```python
from build123d import *

# Parameters (mm, degrees)
BOSS_EXTRUDE1_DEPTH = 165
SKETCH3_W           = 30
SKETCH3_H           = 32
BOSS_EXTRUDE2_DEPTH = 2
SKETCH4_W           = 30
SKETCH4_H           = 32
BOSS_EXTRUDE3_DEPTH = 2
BOSS_EXTRUDE4_START = 10
BOSS_EXTRUDE4_DEPTH = 10
CUT_EXTRUDE1_DEPTH  = 10
BOSS_EXTRUDE6_DEPTH = 15
CUT_EXTRUDE2_DEPTH  = 15
BOSS_EXTRUDE7_DEPTH = 121
CUT_EXTRUDE3_DEPTH  = 121
SKETCH13_W          = 169
SKETCH13_H          = 30
CUT_EXTRUDE5_DEPTH  = 3
SKETCH14_W          = 169
SKETCH14_H          = 30
BOSS_EXTRUDE8_DEPTH = 3
SKETCH12_W          = 28
SKETCH12_H          = 2
CUT_EXTRUDE6_DEPTH  = 168
SKETCH16_W          = 165
SKETCH16_H          = 26
CUT_EXTRUDE7_DEPTH  = 3
CUT_EXTRUDE8_DEPTH  = 1.5
CUT_EXTRUDE9_DEPTH  = 3
SKETCH20_W          = 169
SKETCH20_H          = 30
BOSS_EXTRUDE9_DEPTH = 1
SKETCH21_W          = 165
SKETCH21_H          = 26
CUT_EXTRUDE10_DEPTH = 1
FILLET1_START       = -16
FILLET1_DEPTH       = 35
FILLET1_2_DEPTH     = 32
FILLET2_R           = 1


with BuildPart() as part:
    # Sketch2 → Boss-Extrude1 (new body)
    with BuildSketch(Plane(origin=(0, 0, 0), x_dir=(0, 0, -1), z_dir=(1, 0, 0))):
        with BuildLine():
            Line((-13, 0), (-13, 17))
            Line((-13, 17), (-15, 17))
            Line((-15, 17), (-15, -15))
            Line((-15, -15), (15, -15))
            Line((15, -15), (15, 17))
            Line((15, 17), (13, 17))
            Line((13, 17), (13, 0))
            ThreePointArc((13, 0), (0, -13), (-13, 0))
        make_face()
    extrude(amount=BOSS_EXTRUDE1_DEPTH)

    # Sketch3 → Boss-Extrude2 (add)
    with BuildSketch(Plane(origin=(165, 0, 0), x_dir=(0, 0, -1), z_dir=(1, 0, 0))):
        with Locations((0, 1)):
            Rectangle(SKETCH3_W, SKETCH3_H)
    extrude(amount=BOSS_EXTRUDE2_DEPTH)

    # Sketch4 → Boss-Extrude3 (add)
    with BuildSketch(Plane.ZY):
        with Locations((0, 1)):
            Rectangle(SKETCH4_W, SKETCH4_H)
    extrude(amount=BOSS_EXTRUDE3_DEPTH)

    # Sketch5 → Boss-Extrude4 (add)
    with BuildSketch(Plane.ZY.offset(-165).offset(BOSS_EXTRUDE4_START)):
        with BuildLine():
            Line((-13, 17), (-13, 0))
            ThreePointArc((-13, 0), (0, -13), (13, 0))
            Line((13, 0), (13, 17))
            Line((13, 17), (-13, 17))
        make_face()
    extrude(amount=-BOSS_EXTRUDE4_DEPTH)

    # Sketch6 → Cut-Extrude1 (cut)
    with BuildSketch(Plane.ZY.offset(-155)):
        with BuildLine():
            Line((-2, 0), (-2, 17))
            Line((-2, 17), (2, 17))
            Line((2, 17), (2, 0))
            ThreePointArc((2, 0), (0, -2), (-2, 0))
        make_face()
    extrude(amount=-CUT_EXTRUDE1_DEPTH, mode=Mode.SUBTRACT)

    # Sketch8 → Boss-Extrude6 (add)
    with BuildSketch(Plane(origin=(0, 0, 0), x_dir=(0, 0, -1), z_dir=(1, 0, 0))):
        with BuildLine():
            Line((13, 0), (13, 17))
            Line((13, 17), (-13, 17))
            Line((-13, 17), (-13, 0))
            ThreePointArc((-13, 0), (0, -13), (13, 0))
        make_face()
    extrude(amount=BOSS_EXTRUDE6_DEPTH)

    # Sketch9 → Cut-Extrude2 (cut)
    with BuildSketch(Plane(origin=(15, 0, 0), x_dir=(0, 0, -1), z_dir=(1, 0, 0))):
        with BuildLine():
            Line((-2.125, 0), (-2.125, 17))
            Line((-2.125, 17), (2.125, 17))
            Line((2.125, 17), (2.125, 0))
            ThreePointArc((2.125, 0), (0, -2.125), (-2.125, 0))
        make_face()
    extrude(amount=-CUT_EXTRUDE2_DEPTH, mode=Mode.SUBTRACT)

    # Sketch10 → Boss-Extrude7 (add)
    with BuildSketch(Plane(origin=(15, 0, 0), x_dir=(0, 0, -1), z_dir=(1, 0, 0))):
        with BuildLine():
            Line((13, 0), (13, 17))
            Line((13, 17), (-13, 17))
            Line((-13, 17), (-13, 0))
            ThreePointArc((-13, 0), (0, -13), (13, 0))
        make_face()
    extrude(amount=BOSS_EXTRUDE7_DEPTH)

    # Sketch11 → Cut-Extrude3 (cut)
    with BuildSketch(Plane(origin=(136, 0, 0), x_dir=(0, 0, -1), z_dir=(1, 0, 0))):
        with BuildLine():
            Line((-8.5, 0), (-8.5, 17))
            Line((-8.5, 17), (8.5, 17))
            Line((8.5, 17), (8.5, 0))
            ThreePointArc((8.5, 0), (0, -8.5), (-8.5, 0))
        make_face()
    extrude(amount=-CUT_EXTRUDE3_DEPTH, mode=Mode.SUBTRACT)

    # Sketch13 → Cut-Extrude5 (cut)
    with BuildSketch(Plane(origin=(0, 17, 0), x_dir=(1, 0, 0), z_dir=(0, 1, 0))):
        with Locations((82.5, 0)):
            Rectangle(SKETCH13_W, SKETCH13_H)
    extrude(amount=-CUT_EXTRUDE5_DEPTH, mode=Mode.SUBTRACT)

    # Sketch14 → Boss-Extrude8 (add)
    with BuildSketch(Plane(origin=(0, 14, 0), x_dir=(1, 0, 0), z_dir=(0, 1, 0))):
        with Locations((82.5, 0)):
            Rectangle(SKETCH14_W, SKETCH14_H)
    extrude(amount=BOSS_EXTRUDE8_DEPTH)

    # Sketch12 → Cut-Extrude6 (cut)
    with BuildSketch(Plane(origin=(167, 0, 0), x_dir=(0, 0, -1), z_dir=(1, 0, 0))):
        with Locations((0, 15)):
            Rectangle(SKETCH12_W, SKETCH12_H)
    extrude(amount=-CUT_EXTRUDE6_DEPTH, mode=Mode.SUBTRACT)

    # Sketch16 → Cut-Extrude7 (cut)
    with BuildSketch(Plane(origin=(0, 17, 0), x_dir=(1, 0, 0), z_dir=(0, 1, 0))):
        with Locations((82.5, 0)):
            Rectangle(SKETCH16_W, SKETCH16_H)
    extrude(amount=-CUT_EXTRUDE7_DEPTH, mode=Mode.SUBTRACT)

    # Sketch17 → Cut-Extrude8 (cut)
    with BuildSketch(Plane(origin=(136, 0, 0), x_dir=(0, 0, -1), z_dir=(1, 0, 0))):
        with BuildLine():
            Line((13, 14), (13, 0))
            ThreePointArc((13, 0), (0, -13), (-13, 0))
            Line((-13, 0), (-13, 14))
            Line((-13, 14), (-8.5, 14))
            Line((-8.5, 14), (-8.5, 0))
            ThreePointArc((-8.5, 0), (0, -8.5), (8.5, 0))
            Line((8.5, 0), (8.5, 14))
            Line((8.5, 14), (13, 14))
        make_face()
    extrude(amount=-CUT_EXTRUDE8_DEPTH, mode=Mode.SUBTRACT)

    # Sketch18 → Cut-Extrude9 (cut)
    with BuildSketch(Plane(origin=(15, 0, 0), x_dir=(0, 0, -1), z_dir=(1, 0, 0))):
        with BuildLine():
            Line((8.5, 0), (8.5, 14))
            Line((8.5, 14), (2.125, 14))
            Line((2.125, 14), (2.125, 0))
            ThreePointArc((2.125, 0), (0, -2.125), (-2.125, 0))
            Line((-2.125, 0), (-2.125, 14))
            Line((-2.125, 14), (-8.5, 14))
            Line((-8.5, 14), (-8.5, 0))
            ThreePointArc((-8.5, 0), (0, -8.5), (8.5, 0))
        make_face()
    extrude(amount=-CUT_EXTRUDE9_DEPTH, mode=Mode.SUBTRACT)

    # Sketch20 → Boss-Extrude9 (add)
    with BuildSketch(Plane(origin=(0, 17, 0), x_dir=(1, 0, 0), z_dir=(0, 1, 0))):
        with Locations((82.5, 0)):
            Rectangle(SKETCH20_W, SKETCH20_H)
    extrude(amount=BOSS_EXTRUDE9_DEPTH)

    # Sketch21 → Cut-Extrude10 (cut)
    with BuildSketch(Plane(origin=(0, 18, 0), x_dir=(1, 0, 0), z_dir=(0, 1, 0))):
        with Locations((82.5, 0)):
            Rectangle(SKETCH21_W, SKETCH21_H)
    extrude(amount=-CUT_EXTRUDE10_DEPTH, mode=Mode.SUBTRACT)

    # Fillet1: read off the stored shape, not the designer's step
    # Fillet1 outline → Fillet1 (cut)
    with BuildSketch(Plane(origin=(0, 0, 0), x_dir=(1, 0, 0), z_dir=(0, 1, 0)).offset(FILLET1_START)):
        with BuildLine():
            Line((-2, 15), (-2, 14))
            ThreePointArc((-2, 14), (-1.707106781, 14.707106781), (-1, 15))
            Line((-1, 15), (-2, 15))
        make_face()
        with BuildLine():
            ThreePointArc((-1, -15), (-1.707106781, -14.707106781), (-2, -14))
            Line((-2, -14), (-2, -15))
            Line((-2, -15), (-1, -15))
        make_face()
        with BuildLine():
            Line((167, 15), (166, 15))
            ThreePointArc((166, 15), (166.707106781, 14.707106781), (167, 14))
            Line((167, 14), (167, 15))
        make_face()
        with BuildLine():
            ThreePointArc((167, -14), (166.707106781, -14.707106781), (166, -15))
            Line((166, -15), (167, -15))
            Line((167, -15), (167, -14))
        make_face()
    extrude(amount=FILLET1_DEPTH, mode=Mode.SUBTRACT)

    # Fillet1 2 outline → Fillet1 2 (cut)
    with BuildSketch(Plane.XY.offset(FILLET1_START)):
        with BuildLine():
            Line((167, 18), (166, 18))
            ThreePointArc((166, 18), (166.707106781, 17.707106781), (167, 17))
            Line((167, 17), (167, 18))
        make_face()
        with BuildLine():
            ThreePointArc((-2, 17), (-1.707106781, 17.707106781), (-1, 18))
            Line((-1, 18), (-2, 18))
            Line((-2, 18), (-2, 17))
        make_face()
    extrude(amount=FILLET1_2_DEPTH, mode=Mode.SUBTRACT)

    # Fillet2
    fillet2_edges = [part.edges().sort_by_distance(p)[0] for p in [
        (0, 17, 13),
        (0, 17, -13),
        (165, 17, -13),
        (165, 17, 13),
    ]]
    fillet(fillet2_edges, radius=FILLET2_R)


solid = part.part
```
Here's how the part is built. I have some questions about the finished solid (model axes, mm). A direction names the side the tool comes from. Coordinates: 2 decimals unless noted, no trailing zeros. Order: outer loops, then holes, each group sorted by start corner. A loop starts at its lowest first (then second) coordinate and runs counter-clockwise, first axis right, second up. Notation, with made-up numbers: (-22, 69) - (-17, 69) arc R24 cw to (-17, 88) - close; hole circle Ø3 at (-19.5, 47). An arc over 180 degrees is marked (long way). One line per question, with ' | ' between items.
(1) Will these pins go through, and if not, where does the flat tip stop? pin 1 (1 mm diameter, centred on y = 15, z = -4.5, fed in from +X); pin 2 (8.5 mm diameter, centred on x = 70.5, z = 0, fed in from +Y).
Report:
pin 1: stops at x = -1 | pin 2: stops at y = -7.36
(2) Suppose I cut it at B-B on y = 8. List the corners of the cut face in (x, z) for me (3 decimals), and give its area (3 significant figures).
Report:
outline: (-2, -14) arc R1 ccw to (-1, -15) - (166, -15) arc R1 ccw to (167, -14) - (167, 14) arc R1 ccw to (166, 15) - (-1, 15) arc R1 ccw to (-2, 14) - close; hole (0, -2.125) - (12, -2.125) - (12, -8.5) - (134.5, -8.5) - (134.5, -13) - (155, -13) - (155, -2) - (165, -2) - (165, 2) - (155, 2) - (155, 13) - (134.5, 13) - (134.5, 8.5) - (12, 8.5) - (12, 2.125) - (0, 2.125) - close | area: 2,360 mm2
(3) Suppose I cut it at C-C on x = 18. List the corners of the cut face in (y, z) for me.
Report:
outline: (-15, -15) - (18, -15) - (18, -13) - (16, -13) - (16, -14) - (14, -14) - (14, -8.5) - (0, -8.5) arc R8.5 cw to (0, 8.5) - (14, 8.5) - (14, 14) - (16, 14) - (16, 13) - (18, 13) - (18, 15) - (-15, 15) - close
(4) If we mould it in two halves opening along X, with no side actions, what happens to faces 3 (the flat face through (81, 1, -15)), 4 (the flat face through (155, 1, -3)), 5 (the flat face through (167, -1, 0))? For each: pulls with the +X half, pulls with the -X half, needs draft (parallel to the pull), parting line crosses it, or undercut.
Report:
face 3: needs draft | face 4: undercut | face 5: pulls with the +X half
(5) Suppose I cut it at A-A on z = 0. List the corners of the cut face in (x, y) for me (3 decimals), and give its area (3 significant figures).
Report:
outline: (-2, -15) - (167, -15) - (167, 14) - (165, 14) - (165, -2) - (155, -2) - (155, -13) - (134.5, -13) - (134.5, -8.5) - (12, -8.5) - (12, -2.125) - (0, -2.125) - (0, 14) - (-1, 14) - (-1, 16) - (0, 16) - (0, 18) - (-1, 18) arc R1 ccw to (-2, 17) - close; (165, 16) - (167, 16) - (167, 17) arc R1 ccw to (166, 18) - (165, 18) - close | area: 1,250 mm2
(6) For faces 1 (the flat face through (165, 6, 0)), 2 (the flat face through (84, -15, 0)), which set-ups out of +Z, -Z, +X, -X, +Y, -Y let a thin tool reach every point of the face, with its end or its side?
Report:
face 1: +Y | face 2: +Z, -Z, +X, -X, -Y
(7) Suppose I cut it at D-D on y = -6. List the corners of the cut face in (x, z) for me, and give its area (3 significant figures).
Report:
outline: (-2, -14) arc R1 ccw to (-1, -15) - (166, -15) arc R1 ccw to (167, -14) - (167, 14) arc R1 ccw to (166, 15) - (-1, 15) arc R1 ccw to (-2, 14) - close; hole (12, -6.02) - (134.5, -6.02) - (134.5, -11.53) - (155, -11.53) - (155, 11.53) - (134.5, 11.53) - (134.5, 6.02) - (12, 6.02) - close | area: 3,120 mm2
(8) If I drill on L1, parallel to X at y = 5.5, z = 6.5; L2, parallel to X at y = 7.5, z = 0; L3, parallel to Z at x = 58, y = 4.5, over which ranges is the centre line in solid material (lowest first)?
Report:
L1: x = -2 to 12, 155 to 167 | L2: x = -2 to 0, 165 to 167 | L3: z = -15 to -8.5, 8.5 to 15
